The listing builds one solid part. Answer for the finished solid, in the listing's coordinates (mm). Face numbers are marked on the shaded views. Round coordinates to 2 decimals unless told otherwise and drop trailing zeros. Order: outer loops, then holes, each group sorted by start corner. A loop starts at its lowest first (then second) coordinate and runs counter-clockwise, first axis right, second up. Notation, with made-up numbers: (37.5, -2.75) -> (88.5, -2.75) arc R21 cw to (88.5, 19.25) -> close; hole circle Ø8 at (68.25, -33.75). An arc over 180 degrees is marked (long way). Return JSON: item names as keys, results as strings. Group by question number.
(1) The part is cut by section D-D (y = 12). Determine the outline of the cut face in (x, z).
(2) The part is cut by section C-C (x = 0). Count the separate pieces of the cut face and the enclosed holes in it, plus the area to 3 significant figures.
(3) The part is cut by section B-B (y = 41.6). Determine the outline of the cut face in (x, z).
(4) Consider line 1 (X direction, y = -23, z = 40.4); line 2 (Y direction, x = -23, z = 41.7); line 3 (Y direction, x = 0, z = 40.6) (3 decimals). Determine where each line is inside the solid, lowest interval first. Write a range as [from, to].
(5) The part is cut by section A-A (x = 23). Determine the outline of the cut face in (y, z).
(6) Determine the mould class of the marked faces 1, 2 and 3 for opening direction Y: +Y half, -Y half, draft (parallel to the pull), parting line (faces both ways), or undercut.
(7) Each of these flat-tipped pins is pushed along its axis until it touches: pin 1 (15 mm diameter, centred on x = 0, y = 0, fed in from -Z); pin 2 (4 mm diameter, centred on x = 23, y = 45.35, fed in from -Z); pin 3 (5 mm diameter, centred on x = -10.5, y = 21.5, fed in from -Z); pin 4 (4.5 mm diameter, centred on x = 0, y = 41.6, fed in from -Z). Where does it stop, or does it pass through?
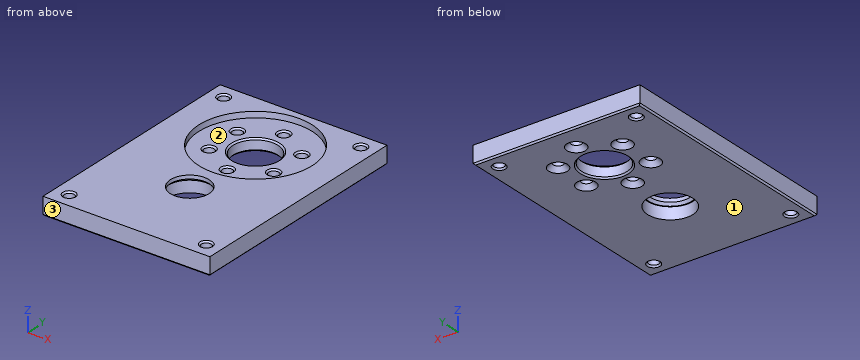
from build123d import *
from OCP.BRepFilletAPI import BRepFilletAPI_MakeChamfer

# Parameters (mm, degrees)
SKETCH1_W                                           = 56
SKETCH1_H                                           = 78.35
SKETCH1_R                                           = 6.5
SKETCH1_R_2                                         = 7.575
BOSS_EXTRUDE1_DEPTH                                 = 5
SKETCH1_4_W                                         = 56
SKETCH1_4_H                                         = 78.35
BOSS_EXTRUDE2_DEPTH                                 = 38
SKETCH4_W                                           = 2
SKETCH4_H                                           = 3
SKETCH7_W                                           = 4.75
SKETCH7_H                                           = 48
BOSS_EXTRUDE3_DEPTH                                 = 15.25
CHAMFER1_SIZE                                       = 17.35
CHAMFER1_SIZE_2                                     = 15.25
SKETCH9_W                                           = 2.7
SKETCH9_H                                           = 5.7
CUT_EXTRUDE11_DEPTH                                 = 8.5
CUT_EXTRUDE12_START                                 = 78.35
SKETCH9_3_W                                         = 2.7
SKETCH9_3_H                                         = 5.7
CUT_EXTRUDE12_DEPTH                                 = 8.5
SKETCH8_R                                           = 1.65
CUT_EXTRUDE5_DEPTH                                  = 175.5
BOSS_EXTRUDE4_START                                 = 38
SKETCH1_5_W                                         = 56
SKETCH1_5_H                                         = 78.35
BOSS_EXTRUDE4_DEPTH                                 = 6
CUT_EXTRUDE2_START                                  = -49
SKETCH2_R                                           = 1.65
CUT_EXTRUDE2_DEPTH                                  = 26
CUT_EXTRUDE6_START                                  = -49
CUT_EXTRUDE6_OUTLINE_R                              = 7.575
CUT_EXTRUDE6_OUTLINE_R_2                            = 6.5
CUT_EXTRUDE6_OUTLINE_R_3                            = 1.65
CUT_EXTRUDE6_DEPTH                                  = 6
CUT_EXTRUDE7_START                                  = -49
SKETCH10_3_R                                        = 19
CUT_EXTRUDE7_DEPTH                                  = 2
CUT_EXTRUDE8_START                                  = -43
SKETCH10_5_R                                        = 7.6
CUT_EXTRUDE8_DEPTH                                  = 4
CUT_EXTRUDE10_START                                 = -6
SKETCH11_2_W                                        = 56
SKETCH11_2_H                                        = 78.35
CUT_EXTRUDE10_DEPTH                                 = 58.25
CSK_FOR_M3_COUNTERSUNK_FLAT_HEAD_SCREW1_D           = 3.4
CSK_FOR_M3_COUNTERSUNK_FLAT_HEAD_SCREW1_DEPTH       = 47
CSK_FOR_M3_COUNTERSUNK_FLAT_HEAD_SCREW1_CSINK_D     = 6.3
CSK_FOR_M3_COUNTERSUNK_FLAT_HEAD_SCREW1_CSINK_ANGLE = 90
CSK_FOR_M3_COUNTERSUNK_FLAT_HEAD_SCREW1_TIP         = 1.021463052
CHAMFER4_SIZE                                       = 0.8
CHAMFER7_SIZE                                       = 0.5


# Read off the part's stored shape, not the designer's step: Cut-Extrude6
with BuildPart() as part:
    # Sketch1 → Boss-Extrude1 (new body)
    with BuildSketch(Plane.XY):
        with Locations((0, 11.175)):
            Rectangle(SKETCH1_W, SKETCH1_H)
        Circle(SKETCH1_R, mode=Mode.SUBTRACT)
        with Locations((0, 29.1)):
            Circle(SKETCH1_R_2, mode=Mode.SUBTRACT)
    extrude(amount=-BOSS_EXTRUDE1_DEPTH)

    # Sketch1<4> → Boss-Extrude2 (add)
    with BuildSketch(Plane.XY):
        with Locations((0, 11.175)):
            Rectangle(SKETCH1_4_W, SKETCH1_4_H)
        with BuildLine():
            ThreePointArc((-9.654082841, 21.972680412), (0, 41.1), (9.654082841, 21.972680412))
            ThreePointArc((9.654082841, 21.972680412), (0, -24), (-9.654082841, 21.972680412))
        make_face(mode=Mode.SUBTRACT)
    extrude(amount=BOSS_EXTRUDE2_DEPTH)

    # Cut-Sweep1: sweep along a path in Sketch3
    with BuildLine(Plane(origin=(0, 0, 38), x_dir=(-1, 0, 0), z_dir=(0, 0, -1))) as cut_sweep1_path:
        Line((26, 0), (26, 26.35))
        ThreePointArc((26, 26.35), (19.556349186, 41.906349186), (4, 48.35))
        Line((4, 48.35), (-4, 48.35))
        ThreePointArc((-4, 48.35), (-19.556349186, 41.906349186), (-26, 26.35))
        Line((-26, 26.35), (-26, -4))
        ThreePointArc((-26, -4), (-19.556349186, -19.556349186), (-4, -26))
        Line((-4, -26), (4, -26))
        ThreePointArc((4, -26), (19.556349186, -19.556349186), (26, -4))
        Line((26, -4), (26, 0))
    # Sketch4 → Cut-Sweep1 (sweep, cut)
    with BuildSketch(Plane(origin=(0, 0, 0), x_dir=(1, 0, 0), z_dir=(0, 1, 0))):
        with Locations((-26, -38.1)):
            Rectangle(SKETCH4_W, SKETCH4_H)
    sweep(path=cut_sweep1_path.line, mode=Mode.SUBTRACT)

    # Sketch7 → Boss-Extrude3 (add)
    with BuildSketch(Plane(origin=(0, 0, -5), x_dir=(-1, 0, 0), z_dir=(0, 0, -1))):
        with Locations((-25.625, 9)):
            Rectangle(SKETCH7_W, SKETCH7_H)
        with Locations((25.625, 9)):
            Rectangle(SKETCH7_W, SKETCH7_H)
    extrude(amount=BOSS_EXTRUDE3_DEPTH)

    # Chamfer1
    chamfer1_edges_1 = [part.edges().sort_by_distance(p)[0] for p in [
        (-25.625, 33, -5),
    ]]
    chamfer1_side_1 = [part.faces().sort_by_distance(p)[0] for p in [
        (-25.625, 33.305, -5),
    ]]
    chamfer1_edges_2 = [part.edges().sort_by_distance(p)[0] for p in [
        (25.625, 33, -5),
    ]]
    chamfer1_side_2 = [part.faces().sort_by_distance(p)[0] for p in [
        (25.625, 33.305, -5),
    ]]
    chamfer1 = BRepFilletAPI_MakeChamfer(part.part.solid().wrapped)
    for e in chamfer1_edges_1:
        chamfer1.Add(CHAMFER1_SIZE - 0.0001, CHAMFER1_SIZE_2 - 0.0001, e.wrapped, chamfer1_side_1[0].wrapped)
    for e in chamfer1_edges_2:
        chamfer1.Add(CHAMFER1_SIZE - 0.0001, CHAMFER1_SIZE_2 - 0.0001, e.wrapped, chamfer1_side_2[0].wrapped)
    add(Compound.cast(chamfer1.Shape()), mode=Mode.REPLACE)  # a hair under: the kernel refuses the full size

    # Sketch9 → Cut-Extrude11 (cut)
    with BuildSketch(Plane(origin=(-22.35, 50.35, 0), x_dir=(0, 0, -1), z_dir=(0, -1, 0))):
        with Locations((-33.65, -0.65)):
            Rectangle(SKETCH9_W, SKETCH9_H)
        with Locations((-33.65, 45.35)):
            Rectangle(SKETCH9_W, SKETCH9_H)
    extrude(amount=CUT_EXTRUDE11_DEPTH, mode=Mode.SUBTRACT)

    # Sketch9<3> → Cut-Extrude12 (cut)
    with BuildSketch(Plane(origin=(-22.35, 50.35, 0), x_dir=(0, 0, -1), z_dir=(0, -1, 0)).offset(CUT_EXTRUDE12_START)):
        with Locations((-33.65, -0.65)):
            Rectangle(SKETCH9_3_W, SKETCH9_3_H)
        with Locations((-33.65, 45.35)):
            Rectangle(SKETCH9_3_W, SKETCH9_3_H)
    extrude(amount=-CUT_EXTRUDE12_DEPTH, mode=Mode.SUBTRACT)

    # Sketch8 → Cut-Extrude5 (cut)
    with BuildSketch(Plane(origin=(28, 0, 0), x_dir=(0, 0, -1), z_dir=(1, 0, 0))):
        with Locations(Location((15.25, -9, 0), (0, 0, 270))):
            Circle(SKETCH8_R)
        with Locations(Location((15.25, 28, 0), (0, 0, 270))):
            Circle(SKETCH8_R)
    extrude(amount=-CUT_EXTRUDE5_DEPTH, mode=Mode.SUBTRACT)

    # Sketch1<5> → Boss-Extrude4 (add)
    with BuildSketch(Plane.XY.offset(BOSS_EXTRUDE4_START)):
        with Locations((0, 11.175)):
            Rectangle(SKETCH1_5_W, SKETCH1_5_H)
    extrude(amount=BOSS_EXTRUDE4_DEPTH)

    # Sketch2 → Cut-Extrude2 (cut)
    with BuildSketch(Plane(origin=(0, 0, -5), x_dir=(-1, 0, 0), z_dir=(0, 0, -1)).offset(CUT_EXTRUDE2_START)):
        with Locations(Location((-23, 45.35, 0), (0, 0, 180))):
            Circle(SKETCH2_R)
        with Locations(Location((23, 45.35, 0), (0, 0, 180))):
            Circle(SKETCH2_R)
        with Locations(Location((-23, -23, 0), (0, 0, 180))):
            Circle(SKETCH2_R)
        with Locations(Location((23, -23, 0), (0, 0, 180))):
            Circle(SKETCH2_R)
    extrude(amount=CUT_EXTRUDE2_DEPTH, mode=Mode.SUBTRACT)

    # Cut-Extrude6 outline → Cut-Extrude6 (cut)
    with BuildSketch(Plane(origin=(0, 0, -5), x_dir=(-1, 0, 0), z_dir=(0, 0, -1)).offset(CUT_EXTRUDE6_START)):
        with Locations((0, 29.1)):
            Circle(CUT_EXTRUDE6_OUTLINE_R)
        Circle(CUT_EXTRUDE6_OUTLINE_R_2)
        with Locations((-10.825317547, 35.35)):
            Circle(CUT_EXTRUDE6_OUTLINE_R_3)
        with Locations((-10.825317547, 22.85)):
            Circle(CUT_EXTRUDE6_OUTLINE_R_3)
        with Locations((0, 16.6)):
            Circle(CUT_EXTRUDE6_OUTLINE_R_3)
        with Locations((10.825317547, 22.85)):
            Circle(CUT_EXTRUDE6_OUTLINE_R_3)
        with Locations((10.825317547, 35.35)):
            Circle(CUT_EXTRUDE6_OUTLINE_R_3)
        with Locations((0, 41.6)):
            Circle(CUT_EXTRUDE6_OUTLINE_R_3)
    extrude(amount=CUT_EXTRUDE6_DEPTH, mode=Mode.SUBTRACT)

    # Sketch10<3> → Cut-Extrude7 (cut)
    with BuildSketch(Plane(origin=(0, 0, -5), x_dir=(-1, 0, 0), z_dir=(0, 0, -1)).offset(CUT_EXTRUDE7_START)):
        with Locations((0, 29.1)):
            Circle(SKETCH10_3_R)
    extrude(amount=CUT_EXTRUDE7_DEPTH, mode=Mode.SUBTRACT)

    # Sketch10<5> → Cut-Extrude8 (cut)
    with BuildSketch(Plane(origin=(0, 0, -5), x_dir=(-1, 0, 0), z_dir=(0, 0, -1)).offset(CUT_EXTRUDE8_START)):
        Circle(SKETCH10_5_R)
    extrude(amount=-CUT_EXTRUDE8_DEPTH, mode=Mode.SUBTRACT)

    # Sketch11<2> → Cut-Extrude10 (cut)
    with BuildSketch(Plane.XY.offset(44).offset(CUT_EXTRUDE10_START)):
        with Locations((0, 11.175)):
            Rectangle(SKETCH11_2_W, SKETCH11_2_H)
    extrude(amount=-CUT_EXTRUDE10_DEPTH, mode=Mode.SUBTRACT)

    # CSK for M3 Countersunk Flat Head Screw1
    with Locations(Plane(origin=(0, 0, 38), x_dir=(-1, 0, 0), z_dir=(0, 0, -1))):
        with Locations((-10.825317547, 35.35), (0, 41.6), (10.825317547, 35.35), (10.825317547, 22.85), (0, 16.6), (-10.825317547, 22.85)):
            CounterSinkHole(CSK_FOR_M3_COUNTERSUNK_FLAT_HEAD_SCREW1_D / 2, CSK_FOR_M3_COUNTERSUNK_FLAT_HEAD_SCREW1_CSINK_D / 2, depth=CSK_FOR_M3_COUNTERSUNK_FLAT_HEAD_SCREW1_DEPTH, counter_sink_angle=CSK_FOR_M3_COUNTERSUNK_FLAT_HEAD_SCREW1_CSINK_ANGLE)
            with Locations((0, 0, -(CSK_FOR_M3_COUNTERSUNK_FLAT_HEAD_SCREW1_DEPTH + CSK_FOR_M3_COUNTERSUNK_FLAT_HEAD_SCREW1_TIP / 2))):  # 118° drill point
                Cone(0, CSK_FOR_M3_COUNTERSUNK_FLAT_HEAD_SCREW1_D / 2, CSK_FOR_M3_COUNTERSUNK_FLAT_HEAD_SCREW1_TIP, mode=Mode.SUBTRACT)

    # Chamfer4
    chamfer4_edges = [part.edges().sort_by_distance(p)[0] for p in [
        (6.5, 0, 42),
    ]]
    chamfer(chamfer4_edges, length=CHAMFER4_SIZE)

    # Chamfer7
    chamfer7_edges = [part.edges().sort_by_distance(p)[0] for p in [
        (-24.65, 45.35, 44),
        (21.35, -23, 44),
        (-24.65, -23, 44),
        (21.35, 45.35, 44),
        (7.575, 29.1, 38),
        (7.575, 29.1, 42),
        (21.35, 45.35, 38),
        (-24.65, -23, 38),
        (21.35, -23, 38),
        (-24.65, 45.35, 38),
        (-28, 11.175, 38),
        (0, -28, 38),
        (28, 11.175, 38),
        (0, 50.35, 38),
        (9.125317547, 22.85, 42),
        (-1.7, 16.6, 42),
        (-12.525317547, 22.85, 42),
        (-12.525317547, 35.35, 42),
        (-1.7, 41.6, 42),
        (9.125317547, 35.35, 42),
    ]]
    chamfer(chamfer7_edges, length=CHAMFER7_SIZE)


solid = part.part
Answer below:
{
 "1": {"outline": "(-28, 38.5) -> (-27.5, 38) -> (27.5, 38) -> (28, 38.5) -> (28, 44) -> (8.28, 44) -> (8.28, 42) -> (-8.28, 42) -> (-8.28, 44) -> (-28, 44) -> close"},
 "2": {"separate pieces": "5", "enclosed holes": "0", "area": "213 mm²"},
 "3": {"outline": "(-28, 38.5) -> (-27.5, 38) -> (-3.15, 38) -> (-1.7, 39.45) -> (-1.7, 41.5) -> (-2.2, 42) -> (-14.31, 42) -> (-14.31, 44) -> (-28, 44) -> close; (1.7, 39.45) -> (3.15, 38) -> (27.5, 38) -> (28, 38.5) -> (28, 44) -> (14.31, 44) -> (14.31, 42) -> (2.2, 42) -> (1.7, 41.5) -> close"},
 "4": {"line 1": "x = [-28, -24.65], [-21.35, 21.35], [24.65, 28]", "line 2": "y = [-28, -24.65], [-21.35, 43.7], [47, 50.35]", "line 3": "y = [-28, -7.6], [7.6, 14.9], [18.3, 21.525], [36.675, 39.9], [43.3, 50.35]"},
 "5": {"outline": "(-28, 38.5) -> (-27.5, 38) -> (-25.15, 38) -> (-24.65, 38.5) -> (-24.65, 43.5) -> (-25.15, 44) -> (-28, 44) -> close; (-21.35, 38.5) -> (-20.85, 38) -> (43.2, 38) -> (43.7, 38.5) -> (43.7, 43.5) -> (43.2, 44) -> (-20.85, 44) -> (-21.35, 43.5) -> close; (47, 38.5) -> (47.5, 38) -> (49.85, 38) -> (50.35, 38.5) -> (50.35, 44) -> (47.5, 44) -> (47, 43.5) -> close"},
 "6": {"face 1": "draft", "face 2": "undercut", "face 3": "-Y half"},
 "7": {"pin 1": "stops at z = 42", "pin 2": "stops at z = 38.15", "pin 3": "stops at z = 38", "pin 4": "stops at z = 38.9"}
}
